Geometry: see drawing. Coordinates: mm, zero at the bounding-box minimum. A direction names the side the tool comes from. Round coordinates to 2 decimals unless told otherwise and drop trailing zeros. Order: outer loops, then holes, each group sorted by start corner. A loop starts at its lowest first (then second) coordinate and runs counter-clockwise, first axis right, second up. Notation, with made-up numbers: (-9, 7) -> (14, 7) arc R7 ccw to (14, 19) -> close; hole circle Ø6 at (-15, 62.5). An arc over 180 degrees is marked (long way). Write item = value, one per line. Start each with the question number.
(1) Cut plane A-A on z = 28.58. Return the cut outline in (x, y), then the cut area to 3 significant figures.
(2) Contact query for flat-ended pins moving along their axis: pin 1 Ø8 at (x, z) = (68, 41) entering from +Y; pin 2 Ø6 at (x, y) = (60, 13) entering from +Z; pin 3 Ø7 at (x, y) = (3.5, 27.5) entering from +Z. Output: stop coordinate, or through.
(3) Cut plane B-B on y = 26. Return the cut outline in (x, z).
(4) Cut plane C-C on z = 43.5. Return the cut outline in (x, y) (1 decimal).
(5) Reachability of the marked faces 1, 2 and 3 from +Z, -Z, +X, -X, +Y, -Y: full face, straight path, thin tool, end or side. Return the list, or none.
(6) Ray query, line 1 (X direction, y = 0.4, z = 11.58); line 2 (X direction, y = 28.5, z = 22); line 3 (X direction, y = 28.25, z = 11.58). Return the intervals inside material, ascending.
(7) Draft query along Y for the marked faces 4, 5 and 6. Return one class per face: released by +Y, released by -Y, zero draft, split by the parting line, or undercut.
(8) Cut plane D-D on y = 5.5. Return the cut outline in (x, z).
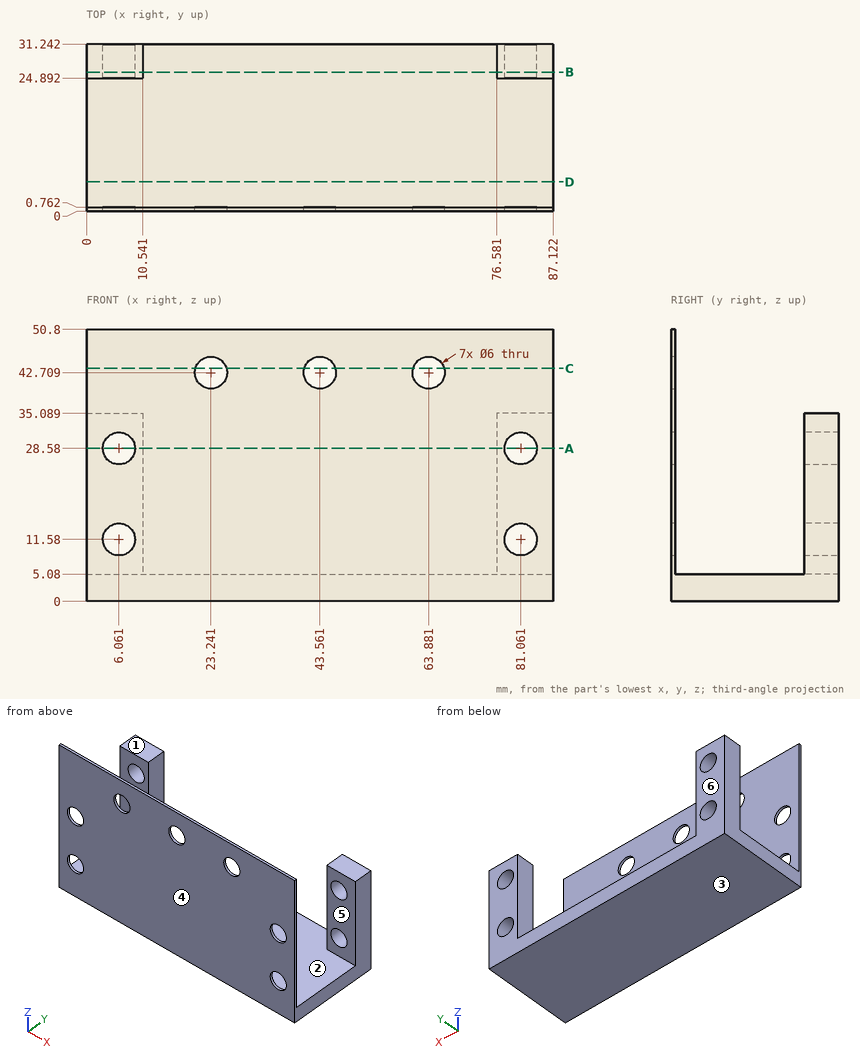
Evaluation:
q1.outline = (0, 0) -> (3.06, 0) -> (3.06, 0.76) -> (0, 0.76) -> close; (0, 24.89) -> (3.06, 24.89) -> (3.06, 31.24) -> (0, 31.24) -> close; (9.06, 0) -> (78.06, 0) -> (78.06, 0.76) -> (9.06, 0.76) -> close; (9.06, 24.89) -> (10.54, 24.89) -> (10.54, 31.24) -> (9.06, 31.24) -> close; (76.58, 24.89) -> (78.06, 24.89) -> (78.06, 31.24) -> (76.58, 31.24) -> close; (84.06, 0) -> (87.12, 0) -> (87.12, 0.76) -> (84.06, 0.76) -> close; (84.06, 24.89) -> (87.12, 24.89) -> (87.12, 31.24) -> (84.06, 31.24) -> close
q1.area = 115 mm^2
q2.pin_1 = 0.76
q2.pin_2 = 5.08
q2.pin_3 = 35.09
q3.outline = (0, 0) -> (87.12, 0) -> (87.12, 35.09) -> (76.58, 35.09) -> (76.58, 5.08) -> (10.54, 5.08) -> (10.54, 35.09) -> (0, 35.09) -> close; hole circle Ø6 at (6.06, 11.58); hole circle Ø6 at (6.06, 28.58); hole circle Ø6 at (81.06, 11.58); hole circle Ø6 at (81.06, 28.58)
q4.outline = (0, 0) -> (20.3, 0) -> (20.3, 0.8) -> (0, 0.8) -> close; (26.1, 0) -> (40.7, 0) -> (40.7, 0.8) -> (26.1, 0.8) -> close; (46.5, 0) -> (61, 0) -> (61, 0.8) -> (46.5, 0.8) -> close; (66.8, 0) -> (87.1, 0) -> (87.1, 0.8) -> (66.8, 0.8) -> close
q5.face_1 = +Z, +X, -X, +Y
q5.face_2 = +Z
q5.face_3 = -Z, +X, -X, +Y, -Y
q6.line_1 = 0 to 3.06, 9.06 to 78.06, 84.06 to 87.12
q6.line_2 = 0 to 10.54, 76.58 to 87.12
q6.line_3 = 0 to 3.06, 9.06 to 10.54, 76.58 to 78.06, 84.06 to 87.12
q7.face_4 = released by -Y
q7.face_5 = undercut
q7.face_6 = released by +Y
q8.outline = (0, 0) -> (87.12, 0) -> (87.12, 5.08) -> (0, 5.08) -> close
